Verification items for the finished model (mm, model axes). Face numbers are marked on the shaded views. A direction names the side the tool comes from. Coordinates: 2 decimals unless noted, no trailing zeros. Order: outer loops, then holes, each group sorted by start corner. A loop starts at its lowest first (then second) coordinate and runs counter-clockwise, first axis right, second up. Notation, with made-up numbers: M 64,50.25 L 75,50.25 A28 ccw 75,83.25 Z; hole C -1.75,42.25 d11. An arc over 180 degrees is marked long. Return JSON: item names as keys, results as strings. Group by question number.
Q1. Access from +Z, -Z, +X, -X, +Y, -Y to the whole of each face (thin tool, end or side, straight path). Record for the marked faces 1 and 2.
Q2. Go/stop test with a flat-tipped pin: pin 1 Ø0.5 at (x, y) = (1.5, 0) entering from -Z. Record where the tip stops, or that it passes through.
Q3. Section check B-B, the plane x = 0. Enter the section's corners in (y, z), then the cut area to 3 significant figures.
Q4. Thickness scan on probe 1 along Z at (x, y) = (0, -1.45); probe 2 along Z at (x, y) = (1.3, 0.1); probe 3 along X at (y, z) = (-1.1, -2). Record the ranges inside material, lowest first.
Q5. Section check D-D, the plane z = 0.5. Enter the section's corners in (x, y).
Q6. Section check A-A, the plane z = -1.5. Enter the section's corners in (x, y).
Q7. Section check C-C, the plane y = -0.9. Enter the section's corners in (x, z), then the cut area to 3 significant figures.
Q8. Mould release check, pull along Z, two halves, no side actions. Record for the marked faces 3, 4 and 5: pulls with the +Z half, pulls with the -Z half, needs draft (parallel to the pull), parting line crosses it, or undercut.
from build123d import *

# Parameters (mm, degrees)
F1_DEPTH = 2.5
F2_R     = 1.5
F3_DEPTH = 5


with BuildPart() as f1:
    # F0 (on Front) → F1 (new body, symmetric)
    with BuildSketch(Plane.XZ):
        with BuildLine():
            ThreePointArc((-1.452369, -3.078081), (0, -1.203081), (1.452369, -3.078081))
            ThreePointArc((1.452369, -3.078081), (0, 0.296919), (-1.452369, -3.078081))
        make_face()
    extrude(amount=F1_DEPTH, both=True)

    # F2 (on Top) → F3 (join)
    with BuildSketch(Plane.XY):
        Circle(F2_R)
    extrude(amount=F3_DEPTH)


solid = f1.part
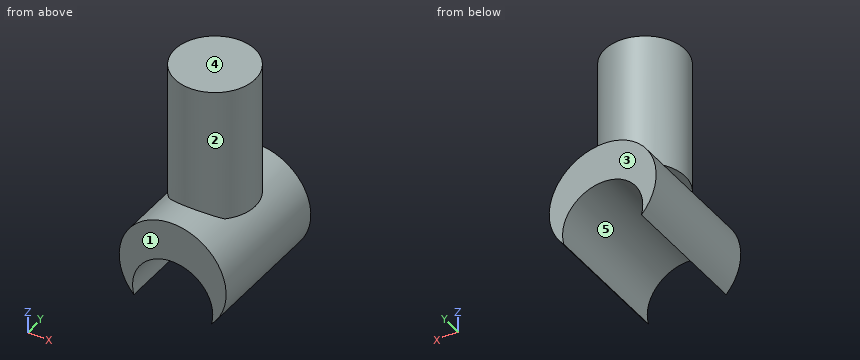
Numbers:
{
 "1": {"face 1": "+Z, -Z, +X, -X, -Y", "face 2": "+Z"},
 "2": {"pin 1": "stops at z = -3.08"},
 "3": {"outline": "M -2.5,-1.2 L 2.5,-1.2 L 2.5,0.3 L 1.5,0.3 L 1.5,5 L -1.5,5 L -1.5,0.3 L -2.5,0.3 Z", "area": "21.6 mm2"},
 "4": {"probe 1": "z = -1.2 to 5", "probe 2": "z = -1.95 to -0.18, 0 to 5", "probe 3": "x = -1.98 to -1.33, 1.33 to 1.98"},
 "5": {"outline": "C 0,0 d3"},
 "6": {"outline": "M -1.99,-2.5 L -0.9,-2.5 L -0.9,2.5 L -1.99,2.5 Z; M 0.9,-2.5 L 1.99,-2.5 L 1.99,2.5 L 0.9,2.5 Z"},
 "7": {"outline": "M -1.45,-3.08 A1.5 cw long 1.45,-3.08 A2 ccw 1.05,0 L 1.2,0 L 1.2,5 L -1.2,5 L -1.2,0 L -1.05,0 A2 ccw Z", "area": "18.2 mm2"},
 "8": {"face 3": "needs draft", "face 4": "pulls with the +Z half", "face 5": "undercut"}
}
